```python
from build123d import *

# Parameters (mm, degrees)
F0_R     = 1.5
F1_DEPTH = 7
F2_SIZE  = 1
F3_R     = 0.5


with BuildPart() as f1:
    # F0 (on Front) → F1 (new body)
    with BuildSketch(Plane.XZ):
        Polygon((0, 7.75), (0, 0), (17, 0), (17, 7.75), (15, 7.75), (2, 7.75), align=None)
        with Locations((5, 4)):
            Circle(F0_R, mode=Mode.SUBTRACT)
        with Locations((12, 4)):
            Circle(F0_R, mode=Mode.SUBTRACT)
        Polygon((0, 15.95), (0, 7.75), (2, 7.75), (2, 13.95), (15, 13.95), (15, 7.75), (17, 7.75), (17, 15.95), align=None)
    extrude(amount=F1_DEPTH)

    # F2
    f2_edges = [f1.edges().sort_by_distance(p)[0] for p in [
        (8.5, 0, 7.75),
        (2, 0, 10.85),
        (8.5, 0, 13.95),
        (15, 0, 10.85),
    ]]
    chamfer(f2_edges, length=F2_SIZE)

    # F3
    f3_edges = [f1.edges().sort_by_distance(p)[0] for p in [
        (8.5, -7, 0),
        (17, -7, 7.975),
        (8.5, -7, 15.95),
        (0, -7, 7.975),
        (17, 0, 7.975),
        (8.5, 0, 0),
        (0, 0, 7.975),
        (8.5, 0, 15.95),
    ]]
    fillet(f3_edges, radius=F3_R)


solid = f1.part
```
Could you check a few things on this model? Use its own coordinates, in mm. A direction names the side the tool comes from. Coordinates: 2 decimals unless noted, no trailing zeros. Write each loop counter-clockwise with the first axis right and the second up, starting at its lowest first coordinate (ties: lowest second). Pieces come first, ordered by that corner, then holes. Notation, with made-up numbers: (-17.5, -3) -> (33.5, -3) arc R18 cw to (33.5, 21) -> close; hole circle Ø11 at (61, 55.5). An arc over 180 degrees is marked (long way). Write item = value, one per line. Start each with the question number.
(1) I want a section at D-D (x = 7). Please give me the cut outline in (y, z), plus the area to 3 significant figures.
(2) We'd pull the mould along X, two halves only. Please class faces 4 (the face through (0, -3, 8)), 5 (the face through (17, -3, 8)), 6 (the face through (15, -4, 11)), 7 (the face through (8, -7, 6)): released by +X, released by -X, zero draft, split by the parting line, or undercut.
(3) I need wall thicknesses on line 1 (Z direction, x = 5, y = -4); line 2 (Z direction, x = 9.5, y = -2.25); line 3 (X direction, y = -4.5, z = 10.5). Which ranges of each line are inside material? Lowest first, please. Write a range as [from, to].
(4) I want a section at A-A (z = 13). Please give me the cut outline in (x, y).
(5) I want a section at C-C (z = 4). Please give me the cut outline in (x, y).
(6) Which directions (+Z, -Z, +X, -X, +Y, -Y) give clear straight access to the entire face, cutting with the end or side of a thin tool? Please do faces 1 (the face through (2, -4, 11)), 2 (the face through (9, -3, 15.95)), 3 (the face through (8.4, -0.49, 14.46)).
(7) I want a section at B-B (x = 5). Please give me the cut outline in (y, z).
Result set:
q1.outline = (-7, 0.5) arc R0.5 ccw to (-6.5, 0) -> (-0.5, 0) arc R0.5 ccw to (0, 0.5) -> (0, 6.75) -> (-1, 7.75) -> (-7, 7.75) -> close; (-7, 13.95) -> (-1, 13.95) -> (0, 14.95) -> (0, 15.45) arc R0.5 ccw to (-0.5, 15.95) -> (-6.5, 15.95) arc R0.5 ccw to (-7, 15.45) -> close
q1.area = 67.0 mm2
q2.face_4 = released by -X
q2.face_5 = released by +X
q2.face_6 = undercut
q2.face_7 = zero draft
q3.line_1 = [0, 2.5], [5.5, 7.75], [13.95, 15.95]
q3.line_2 = [0, 7.75], [13.95, 15.95]
q3.line_3 = [0, 2], [15, 17]
q4.outline = (0, -6.5) arc R0.5 ccw to (0.5, -7) -> (2, -7) -> (2, -1) -> (1, 0) -> (0.5, 0) arc R0.5 ccw to (0, -0.5) -> close; (15, -7) -> (16.5, -7) arc R0.5 ccw to (17, -6.5) -> (17, -0.5) arc R0.5 ccw to (16.5, 0) -> (16, 0) -> (15, -1) -> close
q5.outline = (0, -6.5) arc R0.5 ccw to (0.5, -7) -> (3.5, -7) -> (3.5, 0) -> (0.5, 0) arc R0.5 ccw to (0, -0.5) -> close; (6.5, -7) -> (10.5, -7) -> (10.5, 0) -> (6.5, 0) -> close; (13.5, -7) -> (16.5, -7) arc R0.5 ccw to (17, -6.5) -> (17, -0.5) arc R0.5 ccw to (16.5, 0) -> (13.5, 0) -> close
q6.face_1 = +Y, -Y
q6.face_2 = +Z, +X, -X, +Y, -Y
q6.face_3 = +Y
q7.outline = (-7, 0.5) arc R0.5 ccw to (-6.5, 0) -> (-0.5, 0) arc R0.5 ccw to (0, 0.5) -> (0, 2.5) -> (-7, 2.5) -> close; (-7, 5.5) -> (0, 5.5) -> (0, 6.75) -> (-1, 7.75) -> (-7, 7.75) -> close; (-7, 13.95) -> (-1, 13.95) -> (0, 14.95) -> (0, 15.45) arc R0.5 ccw to (-0.5, 15.95) -> (-6.5, 15.95) arc R0.5 ccw to (-7, 15.45) -> close
